Geometry: final body of the model. Coordinates: model frame, mm. A direction names the side the tool comes from. Coordinates: 2 decimals unless noted, no trailing zeros. Write each loop counter-clockwise with the first axis right and the second up, starting at its lowest first coordinate (ties: lowest second). Pieces come first, ordered by that corner, then holes. Notation, with made-up numbers: (-32, 1.25) -> (22, 1.25) arc R21 ccw to (22, 20.25) -> close; hole circle Ø6 at (69, 64.25). An arc over 180 degrees is marked (long way). One line per item, written item: value.
```python
from build123d import *

# Parameters (mm, degrees)
ESBO_O1_W                = 530
ESBO_O1_H                = 325
RESSALTO_EXTRUS_O1_DEPTH = 15.8
ESBO_O2_W                = 530
ESBO_O2_H                = 25
RESSALTO_EXTRUS_O2_DEPTH = 3.5
ESBO_O3_W                = 530
ESBO_O3_H                = 220
RESSALTO_EXTRUS_O3_DEPTH = 30
CORTE_EXTRUS_O1_DEPTH    = 221
CORTE_EXTRUS_O2_DEPTH    = 221
FILETE2_R                = 10


with BuildPart() as part:
    # Esboço1 → Ressalto-extrusão1 (new body)
    with BuildSketch(Plane.XY):
        with Locations((265, 162.5)):
            Rectangle(ESBO_O1_W, ESBO_O1_H)
    extrude(amount=RESSALTO_EXTRUS_O1_DEPTH)

    # Esboço2 → Ressalto-extrusão2 (add)
    with BuildSketch(Plane.XY.offset(15.8)):
        with Locations((265, 12.5)):
            Rectangle(ESBO_O2_W, ESBO_O2_H)
    extrude(amount=RESSALTO_EXTRUS_O2_DEPTH)

    # Esboço3 → Ressalto-extrusão3 (add)
    with BuildSketch(Plane(origin=(0, 0, 0), x_dir=(-1, 0, 0), z_dir=(0, 0, -1))):
        with Locations((-265, 110)):
            Rectangle(ESBO_O3_W, ESBO_O3_H)
    extrude(amount=RESSALTO_EXTRUS_O3_DEPTH)

    # Esboço4 → Corte-extrusão1 (cut, through all)
    with BuildSketch(Plane(origin=(0, 220, 0), x_dir=(1, 0, 0), z_dir=(0, 1, 0))):
        with BuildLine():
            Line((530, 0), (530, 30))
            Line((530, 30), (420, 30))
            ThreePointArc((420, 30), (448.437782273, 25.577393935), (475, 14.499691353))
            ThreePointArc((475, 14.499691353), (501.560410299, 3.685808879), (530, 0))
        make_face()
    extrude(amount=-CORTE_EXTRUS_O1_DEPTH, mode=Mode.SUBTRACT)

    # Esboço6 → Corte-extrusão2 (cut, through all)
    with BuildSketch(Plane(origin=(0, 220, 0), x_dir=(1, 0, 0), z_dir=(0, 1, 0))):
        with BuildLine():
            Line((0, 0), (0, 30))
            Line((0, 30), (110, 30))
            ThreePointArc((110, 30), (81.495614373, 26.182747301), (55, 15))
            ThreePointArc((55, 15), (28.504385627, 3.817252699), (0, 0))
        make_face()
    extrude(amount=-CORTE_EXTRUS_O2_DEPTH, mode=Mode.SUBTRACT)

    # Filete2
    filete2_edges = [part.edges().sort_by_distance(p)[0] for p in [
        (0, 325, 7.9),
        (530, 325, 7.9),
        (530, 0, 9.65),
        (0, 0, 9.65),
    ]]
    fillet(filete2_edges, radius=FILETE2_R)


solid = part.part
```
(1) Section C-C (z = -6.5). Return the cut outline in (x, y).
Responses:
outline: (36.96, 0) -> (492.48, 0) -> (492.48, 220) -> (36.96, 220) -> close
(2) Section A-A (x = 188.5). Return the cut outline in (y, z).
Responses:
outline: (0, -30) -> (220, -30) -> (220, 0) -> (325, 0) -> (325, 15.8) -> (25, 15.8) -> (25, 19.3) -> (0, 19.3) -> close
(3) Line query: line 1 (Z direction, x = 199, y = 309); line 2 (Y direction, x = 297.5, z = -5.5); line 3 (Z direction, x = 141, y = 165). Output: solid intervals per line, ascending. Write a range as [from, to].
Responses:
line 1: z = [0, 15.8]
line 2: y = [0, 220]
line 3: z = [-30, 15.8]
(4) Reachability of faces 1 (the flat face through (269, 220, -15)), 2 (the flat face through (261, 177, 15.8)), 3 (the flat face through (261, 13, 19.3)) from +Z, -Z, +X, -X, +Y, -Y: full face, straight path, thin tool, end or side. Return the list, or none.
Responses:
face 1: -Z, +X, -X, +Y
face 2: +Z, +X, -X, +Y
face 3: +Z, +X, -X, +Y, -Y
(5) First-contact query: pin 1 (5 mm diameter, centred on x = 290.5, z = -21, fed in from +Y); pin 2 (10 mm diameter, centred on x = 89.5, y = 188.5, fed in from -Z); pin 3 (1.8 mm diameter, centred on x = 319, z = 17.5, fed in from +Y). Flat tips, straight axial feed; report the tip coordinate or a pass-through.
Responses:
pin 1: stops at y = 220
pin 2: stops at z = -28.89
pin 3: stops at y = 25
(6) Section B-B (y = 56). Return the cut outline in (x, z).
Responses:
outline: (0, 0) arc R108.33 cw to (55, -15) arc R108.33 ccw to (110, -30) -> (420, -30) arc R119.79 ccw to (475, -14.5) arc R111.56 cw to (530, 0) -> (530, 15.8) -> (0, 15.8) -> close
(7) Section D-D (y = 299.5). Return the cut outline in (x, z).
Responses:
outline: (0, 0) -> (530, 0) -> (530, 15.8) -> (0, 15.8) -> close
